Here's the drawing with two shaded views (mm, measured from the low corner). I have some questions. A direction names the side the tool comes from. Round coordinates to 2 decimals unless told otherwise and drop trailing zeros. Loops run counter-clockwise (first coordinate to the right, second up) from the corner with the lowest first, then second, coordinate; pieces in that order, holes last.
(1) I want a section at D-D on x = 53. Write out the boundary of the cut face in (y, z).
(2) Which directions (+Z, -Z, +X, -X, +Y, -Y) give clear straight access to the entire face, cutting with the end or side of a thin tool? Please do the marked faces 1 and 2.
(3) Thinking about a two-plate mould opening in X: for the marked faces 3, 4 and 5, which applies, released by +X, released by -X, zero draft, split by the parting line, or undercut?
(4) If I drill on line 1 along Y through (x, z) = (57, 4); line 2 along Y through (x, z) = (46, 2) (1 decimal); line 3 along X through (y, z) = (17.25, 4.25) (1 decimal), over which ranges is the centre line in solid material (lowest first)?
(5) Will this pin go through, and if not, where does the flat tip stop? pin 1 Ø10 at (x, y) = (38, 16) entering from -Z.
(6) I want a section at A-A on y = 19.5. Give the number of separate pieces and of enclosed holes in the cut face, plus the area to 3 significant figures.
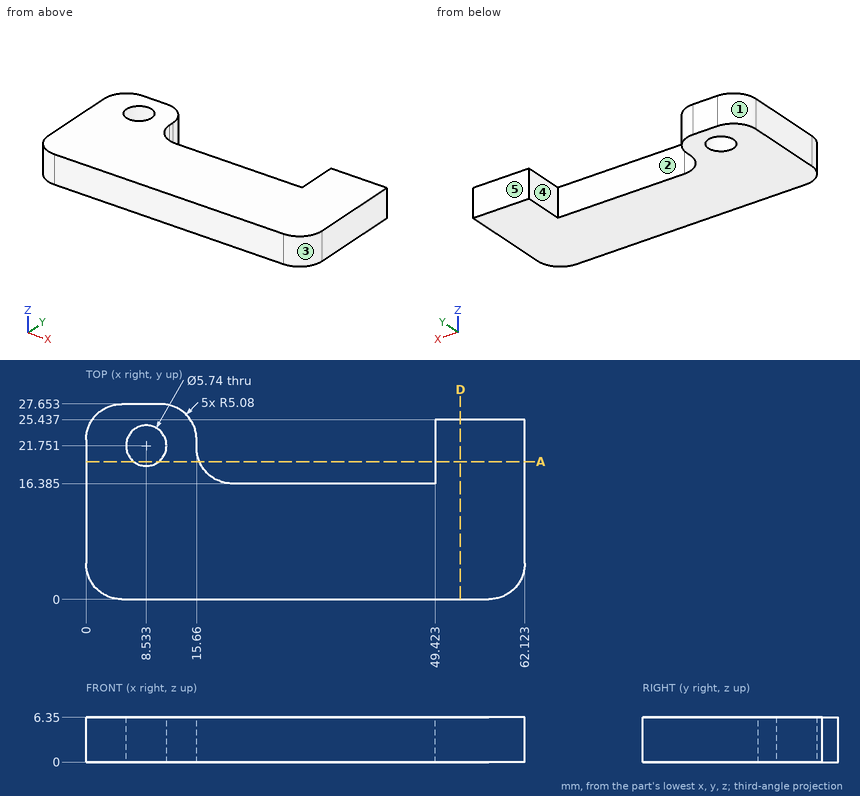
Filled sheet:
1. outline: (0, 0) - (25.44, 0) - (25.44, 6.35) - (0, 6.35) - close
2. face 1: +Z, -Z, -X, +Y
2. face 2: +Z, -Z, +Y
3. face 3: released by +X
3. face 4: undercut
3. face 5: zero draft
4. line 1: y = 0 to 25.44
4. line 2: y = 0 to 16.4
4. line 3: x = 0 to 17.9, 49.4 to 62.1
5. pin 1: stops at z = 0
6. separate pieces: 3
6. enclosed holes: 0
6. area: 160 mm2
